CAD build for the part. Positions are in the model's coordinates, mm. Round coordinates to 2 decimals unless told otherwise and drop trailing zeros. Write each loop counter-clockwise with the first axis right and the second up, starting at its lowest first coordinate (ties: lowest second). Pieces come first, ordered by that corner, then holes. Notation, with made-up numbers: (38, -39) -> (77, -39) arc R15 cw to (77, -10) -> close; hole circle Ø3 at (87, 65.5). An arc over 180 degrees is marked (long way). Answer in a Markdown table with one row per item. Add a question column.
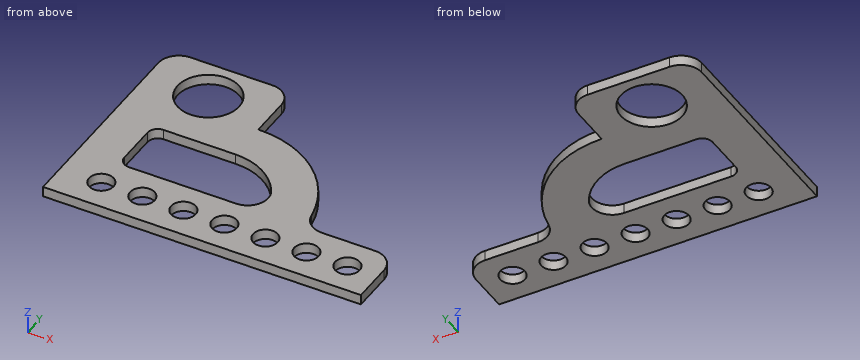
```python
from build123d import *

# Parameters (mm, degrees)
SKETCH2_R           = 15
SKETCH2_R_2         = 6
BOSS_EXTRUDE1_DEPTH = 5


with BuildPart() as part:
    # Sketch2 → Boss-Extrude1 (new body)
    with BuildSketch(Plane.XY):
        with BuildLine():
            Line((0, 0), (-155, 0))
            Line((-155, 0), (-155, 100))
            ThreePointArc((-155, 100), (-152.071067812, 107.071067812), (-145, 110))
            Line((-145, 110), (-105, 110))
            ThreePointArc((-105, 110), (-97.928932188, 107.071067812), (-95, 100))
            Line((-95, 100), (-95, 80))
            ThreePointArc((-95, 80), (-62.725138782, 68.188130791), (-45.699335141, 38.333333333))
            ThreePointArc((-45.699335141, 38.333333333), (-42.294174413, 32.362373842), (-35.839202169, 30))
            Line((-35.839202169, 30), (-10, 30))
            ThreePointArc((-10, 30), (-2.928932188, 27.071067812), (0, 20))
            Line((0, 20), (0, 0))
        make_face()
        with Locations((-125, 90)):
            Circle(SKETCH2_R, mode=Mode.SUBTRACT)
        with Locations((-135, 15)):
            Circle(SKETCH2_R_2, mode=Mode.SUBTRACT)
        with Locations((-115, 15)):
            Circle(SKETCH2_R_2, mode=Mode.SUBTRACT)
        with Locations((-95, 15)):
            Circle(SKETCH2_R_2, mode=Mode.SUBTRACT)
        with Locations((-75, 15)):
            Circle(SKETCH2_R_2, mode=Mode.SUBTRACT)
        with Locations((-55, 15)):
            Circle(SKETCH2_R_2, mode=Mode.SUBTRACT)
        with Locations((-35, 15)):
            Circle(SKETCH2_R_2, mode=Mode.SUBTRACT)
        with Locations((-15, 15)):
            Circle(SKETCH2_R_2, mode=Mode.SUBTRACT)
        with BuildLine():
            Line((-95, 60), (-130, 60))
            ThreePointArc((-130, 60), (-133.535533906, 58.535533906), (-135, 55))
            Line((-135, 55), (-135, 35))
            ThreePointArc((-135, 35), (-133.535533906, 31.464466094), (-130, 30))
            Line((-130, 30), (-95, 30))
            Line((-95, 30), (-77.679491924, 30))
            ThreePointArc((-77.679491924, 30), (-69.019237886, 35), (-69.019237886, 45))
            ThreePointArc((-69.019237886, 45), (-80, 55.980762114), (-95, 60))
        make_face(mode=Mode.SUBTRACT)
    extrude(amount=BOSS_EXTRUDE1_DEPTH)


solid = part.part
```
Item 1: Pin check, flat tips, straight feed: pin 1 (2.5 mm diameter, centred on x = -28, z = 2.5, fed in from +Y); pin 2 (2 mm diameter, centred on y = 48, z = 1.5, fed in from +X); pin 3 (2.5 mm diameter, centred on y = 43, z = 1.5, fed in from +X). Stop position of each tip, or through.
Item 2: Saw through at D-D on y = 90. Give the cut face in (x, z), then the cut area to 3 significant figures.
Item 3: Saw through at A-A on x = -55. Give the cut face in (y, z), then the cut area to 3 significant figures.
Item 4: Saw through at B-B on z = 1.9. Count the separate pieces of the cut face and the enclosed holes in it, then the cut area to 3 significant figures.
Item 5: Drill centre lines: probe 1 along Y at (x, z) = (-90, 3.9); probe 2 along Y at (x, z) = (-115, 1.5); probe 3 along Y at (x, z) = (-75, 3). Where is each one in solid material? Low to high.
Recorded:
| question | item | result |
|---|---|---|
| 1 | pin 1 | y = 30 |
| 1 | pin 2 | x = -47.98 |
| 1 | pin 3 | x = -46.4 |
| 2 | outline | (-155, 0) -> (-140, 0) -> (-140, 5) -> (-155, 5) -> close; (-110, 0) -> (-95, 0) -> (-95, 5) -> (-110, 5) -> close |
| 2 | area | 150 mm2 |
| 3 | outline | (0, 0) -> (9, 0) -> (9, 5) -> (0, 5) -> close; (21, 0) -> (60, 0) -> (60, 5) -> (21, 5) -> close |
| 3 | area | 240 mm2 |
| 4 | separate pieces | 1 |
| 4 | enclosed holes | 9 |
| 4 | area | 8,020 mm2 |
| 5 | probe 1 | 0 to 11.68, 18.32 to 30, 59.58 to 79.75 |
| 5 | probe 2 | 0 to 9, 21 to 30, 60 to 78.82, 101.18 to 110 |
| 5 | probe 3 | 0 to 9, 21 to 30.37, 52.36 to 75.83 |
